Design review of the part built by this model. Coordinates are the model's own, in mm. Face numbers are marked on the shaded views. A direction names the side the tool comes from. Round coordinates to 2 decimals unless told otherwise and drop trailing zeros. Loops run counter-clockwise (first coordinate to the right, second up) from the corner with the lowest first, then second, coordinate; pieces in that order, holes last. Notation, with made-up numbers: (5, -7.5) -> (35, -7.5) arc R24 ccw to (35, 28.5) -> close; hole circle Ø7 at (63, -25.75). An arc over 180 degrees is marked (long way). Answer as CSV lines item,"result". Start each with the question number.
(1) To check wall thickness, follow line 1 (Z direction, x = 5.5, y = -0.5); line 2 (Z direction, x = 11, y = 23); line 3 (Z direction, x = 8.75, y = 23.5). State the ranges of each line that lie inside material, in increasing order. Write a range as from..to.
(2) Machinability: for the marked faces 1, 2, 3 and 4, which of the approach directions +Z, -Z, +X, -X, +Y, -Y give a long, thin tool a straight path to every point of the face, cutting with its end or side? Answer none if there is none.
(3) For P1, Ø3, axis at x = 2, y = 0.5, coming from the -Z side; P2, Ø2.5, axis at y = 22.98, z = 6.5, coming from the -X side; P3, Ø6, axis at y = 3, z = -5, coming from the -X side; P4, Ø1.5, axis at x = 7, y = 19.5, coming from the +Z side, all flat-tipped, find the tip position at first contact; note any pin that passes through.
(4) Take a section at B-B, the plane x = 3.5. Write out the cut boundary in (y, z), and give its area (3 significant figures).
(5) Take a section at D-D, the plane x = 1. Write out the cut boundary in (y, z), and give its area (3 significant figures).
(6) Take a section at A-A, the plane z = -8.5. Write out the cut boundary in (x, y), and give its area (3 significant figures).
(7) Draft analysis for pull direction X (two halves, no side actions). For the marked faces 5, 6, 7 and 8, state which applies: +X half, -X half, draft (parallel to the pull), parting line (faces both ways), or undercut.
(8) Take a section at C-C, the plane y = -3. Write out the cut boundary in (x, z).
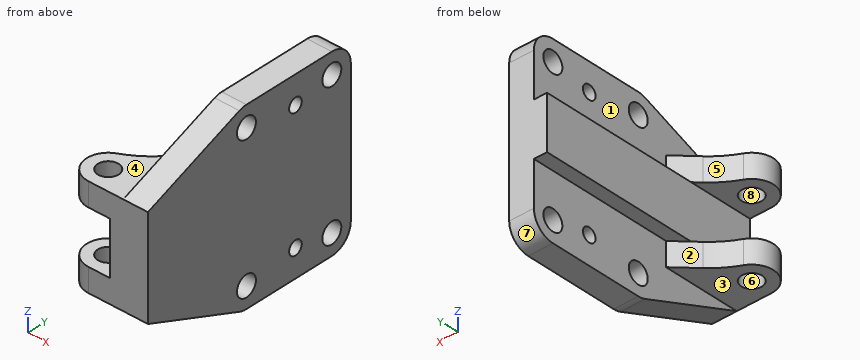
Autodesk Inventor part; units mm, degrees
ref_plane "Work Plane1" through (-0.6712, -8.5, -7.5) normal (0, 0, -1) x (0, 1, 0)
ref_plane "Work Plane2" through (11.5705, 1.2284, -16.2496) normal (-1, 0, 0) x (0, 0, 1)
ref_plane "YZ Plane" through (0, 0, 0) normal (1, 0, 0) x (0, 1, 0)
sketch "Sketch1" plane through (0, 0, 0) normal (0, 0, 1) x (1, 0, 0)
  circle A0 centre (3, -3) radius 1.5
  arc A1 (4.6242, -5.5223) -> (3, 0) centre (3, -3) ccw
  arc A2 (4.6783, -5.6064) -> (3, 0.1) centre (3, -3) ccw
  circle A3 centre (3, -3) radius 3.1
  point P0 (0, 0)
  point P1 (3, 0.1)
  dimension "d0" = 0.1
extrude "Extrusion1" add sketch "Sketch1" along normal blind 3.5
sketch "Sketch2" plane through (3, -3, 0) normal (0, 0, -1) x (-1, 0, 0)
  circle A0 centre (0, 0) radius 3.1
  point P0 (3, 3)
extrude "Extrusion2" cut sketch "Sketch2" against normal blind 0.1
sketch "Sketch3" plane through (3, -3, 3.5) normal (0, 0, 1) x (1, 0, 0)
  circle A0 centre (0, 0) radius 3.1
  line L0 (0, 3.1) -> (5, 3.1)
  line L1 (0, -3.1) -> (5, -3.1)
  line L2 (5, -3.1) -> (5, 3.1)
  point P0 (-3, 3)
  dimension "d5" = 5
  dimension "d6" = 5
ref_plane "Work Plane1" through (-0.6712, -8.5, -7.5) normal (0, 0, -1) x (0, 1, 0)
extrude "Extrusion3" add sketch "Sketch3" against normal up to surface (11 mm away) contours A0 L0 L2 L1
sketch "Sketch4" plane through (8, 0.1, -7.5) normal (0, 0, -1) x (-1, 0, 0)
  arc A0 (5, 0) -> (5, -6.2) centre (5, -3.1) ccw
  line L0 (0, 0) -> (5, 0)
  line L1 (0, -6.2) -> (0, 0)
  line L2 (5, -6.2) -> (0, -6.2)
  point P0 (8, -0.1)
extrude "Extrusion4" add sketch "Sketch4" along normal blind 0.1
sketch "Sketch5" plane through (8, 0.1, -7.6) normal (0, 0, -1) x (-1, 0, 0)
  arc A0 (5, -6.2) -> (5, 0) centre (5, -3.1) ccw
  line L0 (5, -6.2) -> (0, -6.2)
  line L1 (0, -6.2) -> (0, 0)
  line L2 (0, 0) -> (5, 0)
  circle A1 centre (5, -3.1) radius 1.5
  point P0 (8, -0.1)
extrude "Extrusion5" add sketch "Sketch5" along normal blind 3.4
sketch "Sketch6" plane through (3, 0.1, 3.5) normal (0, 1, 0) x (1, 0, 0)
  line L0 (0, 3.5) -> (3, 3.5)
  line L1 (0, 11.1) -> (3.1, 11.1)
  line L2 (0, 3.4) -> (0, 11.1)
  line L3 (0, 3.4) -> (3.1, 3.4)
  line L4 (3.1, 3.4) -> (0, 3.4)
  line L5 (0, 3.4) -> (0, 11.1)
  line L6 (0, 11.1) -> (3.1, 11.1)
  line L7 (3.1, 11.1) -> (3.1, 3.4)
  point P0 (-3, 3.5)
extrude "Extrusion6" cut sketch "Sketch6" against normal through all
sketch "Sketch7" plane through (8, -6.1, 3.5) normal (1, 0, 0) x (0, 0, -1)
  line L0 (0, 0) -> (14.5, 0)
  line L1 (7.25, 0) -> (7.25, 35.3128)
  line L2 (7.25, 0) -> (42.5628, 0) construction
  point P0 (3.5, 6.1)
  dimension "d15" = 90
sketch "Sketch8" plane through (8, -6.1, 3.5) normal (1, 0, 0) x (0, 0, -1)
  circle A0 centre (-3.0004, 15.5784) radius 1.1
  circle A1 centre (-3.0004, 29.0784) radius 1.1
  circle A2 centre (17.4996, 29.0784) radius 1.1
  circle A3 centre (17.4996, 15.5784) radius 1.1
  circle A4 centre (-3.0004, 15.5784) radius 1.5
  circle A5 centre (-3.0004, 29.0784) radius 1.5
  circle A6 centre (17.4996, 29.0784) radius 1.5
  circle A7 centre (17.4996, 15.5784) radius 1.5
  circle A8 centre (17.4996, 15.5784) radius 3
  circle A9 centre (17.4996, 29.0784) radius 3
  circle A10 centre (-3.0004, 29.0784) radius 3
  circle A11 centre (-3.0004, 15.5784) radius 3
  line L0 (-3.0004, 32.0784) -> (17.4996, 32.0784)
  line L1 (-6.0004, 29.0784) -> (-6.0004, 15.5784)
  line L2 (20.4996, 29.0784) -> (20.4996, 15.5784)
  line L3 (-3.0004, 12.5784) -> (17.4996, 12.5784)
  line L4 (0, 6.2) -> (14.5, 6.2)
  line L5 (0, 0) -> (0, 6.2)
  line L6 (0, 0) -> (14.5, 0)
  line L7 (14.5, 6.2) -> (14.5, 0)
  line L8 (0, 0) -> (-5.7858, 14.4642)
  line L9 (14.5, 0) -> (20.2851, 14.4643)
  point P0 (3.5, 6.1)
  dimension "d16" = 3
  dimension "d17" = 3
  dimension "d18" = 3
  dimension "d19" = 3
  dimension "d20" = 6
  dimension "d21" = 6
  dimension "d22" = 6
  dimension "d23" = 6
ref_plane "Work Plane2" through (11.5705, 1.2284, -16.2496) normal (-1, 0, 0) x (0, 0, 1)
extrude "Extrusion7" add sketch "Sketch8" along normal up to surface (3.5705 mm away) contours A8 | A8 L3 A11 L1 A10 L0 A9 L2 | A8 L9 L7 L4 L5 L8 A11 L3 | A9 | A11 | L6 L5 L4 L7 | A10
sketch "Sketch9" plane through (3, 0.1, 3.5) normal (0, 1, 0) x (1, 0, 0)
  line L0 (3.1, 11.1) -> (3.1, 3.4)
  line L1 (5, 17.4996) -> (5, -3.0004)
  line L2 (3.1, 11.1) -> (0, 11.1)
  line L3 (3.1, 11.1) -> (5, 11.1)
  line L4 (5, 11.1) -> (5, 3.4)
  line L5 (5, 3.4) -> (3.1, 3.4)
  line L6 (3.1, 3.4) -> (3.1, 11.1)
  point P0 (-3, 3.5)
  point P1 (3.1, 3.4)
  point P2 (5, 11.1)
extrude "Extrusion8" add sketch "Sketch9" along normal up to surface (25.8784 mm away)
sketch "Sketch10" plane through (11.5705, 9.4784, -16.9996) normal (1, 0, 0) x (0, 0, -1)
  circle A0 centre (-22.5, 7.75) radius 0.5
  circle A1 centre (-4, 7.75) radius 0.5
  circle A2 centre (-22.5, 7.75) radius 1
  circle A3 centre (-4, 7.75) radius 1
  point P0 (-16.9996, -9.4784)
  dimension "d29" = 2
  dimension "d30" = 2
extrude "Extrusion9" cut sketch "Sketch10" against normal through all contours A0 | A1 | A2 | A3
chamfer "Chamfer1" distance 5 angle 45 2 edges at (8, 0.1, 1.8) (8, 0.1, -9.3)
fillet "Fillet1" radius 13 2 edges at (3, 0.1, -9.3) (3, 0.1, 1.8)
properties part number "TheCamera_3DPrint"
The answers:
1,line 1,"-11..-7.6, 0.1..3.5"
1,line 2,"-17..-15.5, -12.5..5, 8..9.5"
1,line 3,"-16.95..-15.41, -12.59..5.09, 7.91..9.45"
2,face 1,"+Z, -X, +Y"
2,face 2,"-Z, -X, +Y"
2,face 3,"-Z, -X, +Y, -Y"
2,face 4,"+Z, -X, +Y, -Y"
3,P1,"z = -11"
3,P2,"through"
3,P3,"x = 4.32"
3,P4,"z = 0.1"
4,outline,"(-6.1, -11) -> (-4.41, -11) -> (-4.41, -7.6) -> (-6.1, -7.6) -> close; (-6.1, 0.1) -> (-4.41, 0.1) -> (-4.41, 3.5) -> (-6.1, 3.5) -> close; (-1.59, -11) -> (0.87, -11) -> (0.87, -7.6) -> (-1.59, -7.6) -> close; (-1.59, 0.1) -> (0.87, 0.1) -> (0.87, 3.5) -> (-1.59, 3.5) -> close"
4,area,"28.2 mm²"
5,outline,"(-5.37, -11) -> (-0.63, -11) -> (-0.63, -7.6) -> (-5.37, -7.6) -> close; (-5.37, 0.1) -> (-0.63, 0.1) -> (-0.63, 3.5) -> (-5.37, 3.5) -> close"
5,area,"32.2 mm²"
6,outline,"(1.66, -0.21) arc R3.1 ccw to (3, -6.1) -> (11.57, -6.1) -> (11.57, 25.98) -> (8, 25.98) -> (8, 5.1) -> (5.22, 2.32) arc R13 cw to start; hole circle Ø3 at (3, -3)"
6,area,"167 mm²"
7,face 5,"-X half"
7,face 6,"undercut"
7,face 7,"draft"
7,face 8,"undercut"
8,outline,"(-0.1, -11) -> (1.5, -11) -> (1.5, -7.6) -> (-0.1, -7.6) -> close; (-0.1, 0.1) -> (1.5, 0.1) -> (1.5, 3.5) -> (-0.1, 3.5) -> close; (4.5, -11) -> (8, -11) -> (8, -12.24) -> (11.57, -12.24) -> (11.57, 4.74) -> (8, 4.74) -> (8, 3.5) -> (4.5, 3.5) -> (4.5, 0.1) -> (6.1, 0.1) -> (6.1, -7.6) -> (4.5, -7.6) -> close"
